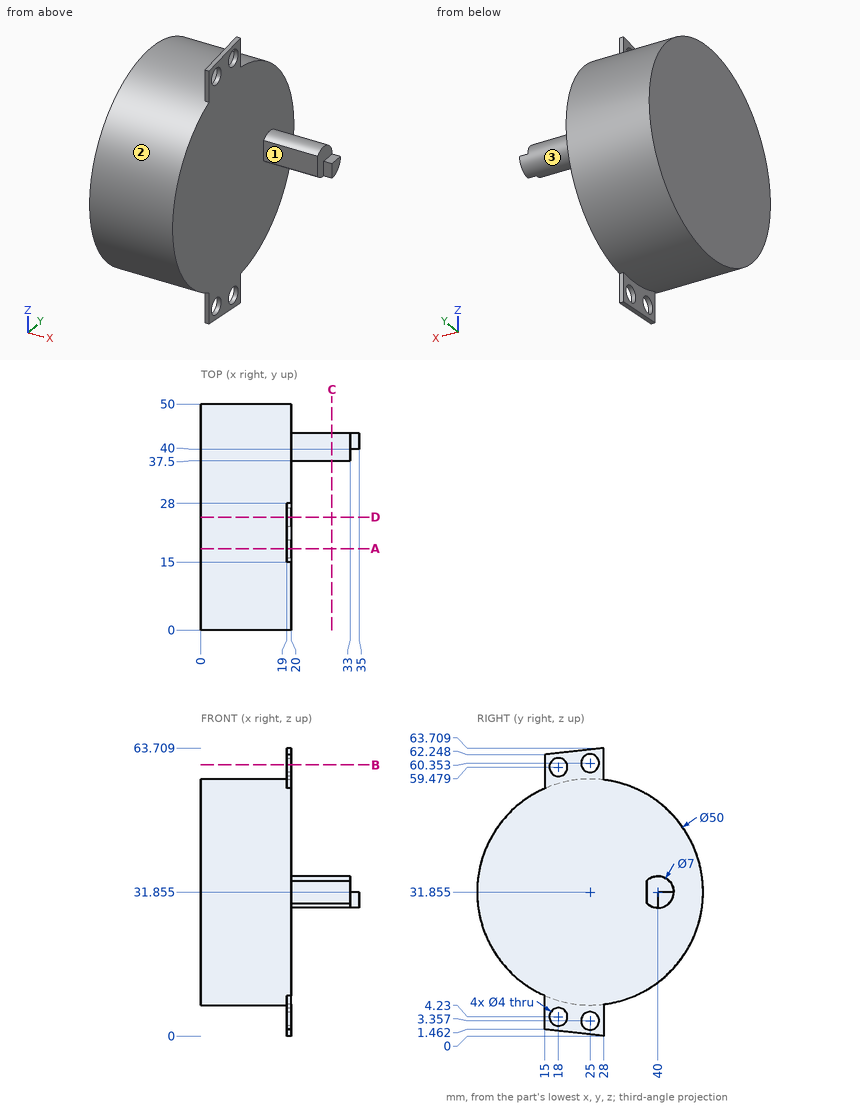
Design review of the part shown in the three views and the two pictorial views. Dimensions are in mm from the part's minimum x, y and z. A direction names the side the tool comes from. Round coordinates to 2 decimals unless told otherwise and drop trailing zeros. Write each loop counter-clockwise with the first axis right and the second up, starting at its lowest first coordinate (ties: lowest second). Pieces come first, ordered by that corner, then holes. Notation, with made-up numbers: (41.5, -1) - (89.5, -1) arc R29 cw to (89.5, 25) - close; hole circle Ø1 at (50, 63). An arc over 180 degrees is marked (long way). Write item = value, one per line. Start each with the question number.
1. Consider section C-C on x = 29. State the section outline as (y, z) points (1 decimal), plus the area to 3 significant figures.
2. Consider section D-D on y = 25. State the section outline as (x, z) points (1 decimal), plus the area to 4 significant figures.
3. Wall thickness on L1, parallel to X at y = 19, z = 21.5; L2, parallel to Y at x = 11, z = 31 (1 decimal); L3, parallel to Z at x = 10, y = 42 (1 decimal): over which ranges is each line inside the solid? List them lowest first.
4. Consider section A-A on y = 18. State the section outline as (x, z) points (1 decimal).
5. For pin 1 Ø3.5 at (y, z) = (18, 4.23) entering from +X; pin 2 Ø8 at (x, z) = (23, 48.5) entering from +Y; pin 3 Ø4.5 at (y, z) = (25, 60.35) entering from -X; pin 4 Ø1 at (x, z) = (11, 44.5) entering from -Y, all flat-tipped, find the tip position at first contact; note any pin that passes through.
6. For the marked faces 1, 2 and 3, list the 3-axis set-ups (+Z, -Z, +X, -X, +Y, -Y) from which the entire face can be reached by the end or side of a thin tool; tool diameter is ignored.
7. Consider section B-B on z = 60. State the section outline as (x, y) points.
Evaluation:
q1.outline = (37.5, 29.4) arc R3.5 ccw (long way) to (37.5, 34.3) - close
q1.area = 35.1 mm2
q2.outline = (0, 6.9) - (19, 6.9) - (19, 5.4) - (20, 5.4) - (20, 58.4) - (19, 58.4) - (19, 56.9) - (0, 56.9) - close; (19, 0.3) - (20, 0.3) - (20, 1.4) - (19, 1.4) - close; (19, 62.4) - (20, 62.4) - (20, 63.4) - (19, 63.4) - close
q2.area = 1,005 mm2
q3.L1 = 0 to 20
q3.L2 = 0 to 50
q3.L3 = 13.5 to 50.2
q4.outline = (0, 7.9) - (19, 7.9) - (19, 6.2) - (20, 6.2) - (20, 57.5) - (19, 57.5) - (19, 55.9) - (0, 55.9) - close; (19, 1.1) - (20, 1.1) - (20, 2.2) - (19, 2.2) - close; (19, 61.5) - (20, 61.5) - (20, 62.6) - (19, 62.6) - close
q5.pin_1 = through
q5.pin_2 = 45.71
q5.pin_3 = 19
q5.pin_4 = 3.15
q6.face_1 = +Z, -Z, +X, -Y
q6.face_2 = -X
q6.face_3 = +X
q7.outline = (19, 15) - (20, 15) - (20, 16.07) - (19, 16.07) - close; (19, 19.93) - (20, 19.93) - (20, 23.03) - (19, 23.03) - close; (19, 26.97) - (20, 26.97) - (20, 28) - (19, 28) - close
